Build history of the part. All positions in model axes, mm. A direction names the side the tool comes from. Give positions to 0.01 mm unless a question says otherwise; leave off trailing zeros. Write each loop counter-clockwise with the first axis right and the second up, starting at its lowest first coordinate (ties: lowest second). Pieces come first, ordered by that corner, then holes. Notation, with made-up numbers: (55.25, 47) -> (99.25, 47) arc R16 ccw to (99.25, 61) -> close; hole circle Ø11 at (-6, 75). An arc over 180 degrees is marked (long way). One line per question, with ' | ' between items. Start each with the question number.
(1) Tool access for faces 1 (the cylindrical face through (4.93, 9.352, -9.474)), 2 (the flat face through (0, 0.2, -3.3)): list every direction of +Z, -Z, +X, -X, +Y, -Y with a clear straight run to the whole face (end or side of a thin tool).
(2) Band-saw the part on C-C, the plane x = 86.5. Give the cut face in (y, z).
(3) Drill centre lines: probe 1 along Y at (x, z) = (6.25, -8); probe 2 along Y at (x, z) = (0.7, 0); probe 3 along X at (y, z) = (8.5, -14). Where is each one in solid material? Low to high. Write a range as from..to.
(4) Pin check, flat tips, straight feed: P1, Ø5, axis at x = 73.5, y = -7.5, coming from the -Z side; P2, Ø10, axis at x = 72, z = -0.5, coming from the -Y side; P3, Ø1.5, axis at x = 111.5, y = 2.5, coming from the +Z side; P4, Ø1.5, axis at y = -15, z = -14, coming from the -X side. Stop position of each tip, or through.
(5) Pull direction Z, two halves, no side cores. Call faces 3 (the flat face through (123.8, 0, 0)), 4 (the flat face through (10, -8, -8)), 5 (the cylindrical face through (87.16, 18.59, 2.44)): released by +Z, released by -Z, zero draft, split by the parting line, or undercut.
from build123d import *

# Parameters (mm, degrees)
SKETCH2_R           = 16
BOSS_EXTRUDE1_DEPTH = 48.8
SKETCH3_R           = 18.75
BOSS_EXTRUDE2_DEPTH = 75
FILLET1_R           = 2.74
SKETCH4_R           = 3
CUT_EXTRUDE1_DEPTH  = 2
SKETCH5_R           = 2
CUT_EXTRUDE2_DEPTH  = 10


with BuildPart() as part:
    # Sketch2 → Boss-Extrude1 (new body)
    with BuildSketch(Plane(origin=(0, 0, 0), x_dir=(0, 0, -1), z_dir=(1, 0, 0))):
        Circle(SKETCH2_R)
    extrude(amount=BOSS_EXTRUDE1_DEPTH)

    # Sketch3 → Boss-Extrude2 (add)
    with BuildSketch(Plane(origin=(48.8, 0, 0), x_dir=(0, 0, -1), z_dir=(1, 0, 0))):
        Circle(SKETCH3_R)
    extrude(amount=BOSS_EXTRUDE2_DEPTH)

    # Fillet1
    fillet1_edges = [part.edges().sort_by_distance(p)[0] for p in [
        (48.8, 0, 18.75),
    ]]
    fillet(fillet1_edges, radius=FILLET1_R)

    # Sketch4 → Cut-Extrude1 (cut)
    with BuildSketch(Plane.ZY):
        Circle(SKETCH4_R)
    extrude(amount=-CUT_EXTRUDE1_DEPTH, mode=Mode.SUBTRACT)

    # Sketch5 → Cut-Extrude2 (cut)
    with BuildSketch(Plane.ZY):
        with Locations((-8, 8)):
            Circle(SKETCH5_R)
        with Locations(Location((8, 8, 0), (0, 0, 180))):
            Circle(SKETCH5_R)
        with Locations((8, -8)):
            Circle(SKETCH5_R)
        with Locations(Location((-8, -8, 0), (0, 0, 180))):
            Circle(SKETCH5_R)
    extrude(amount=-CUT_EXTRUDE2_DEPTH, mode=Mode.SUBTRACT)


solid = part.part
Results:
1) face 1: -X | face 2: +Z, -Z, -X, +Y, -Y
2) outline: circle Ø37.5 at (0, 0)
3) probe 1: y = -13.86..-10, -6..6, 10..13.86 | probe 2: y = -16..-3, 3..16 | probe 3: x = 48.82..123.8
4) P1: stops at z = -18.07 | P2: stops at y = -18.75 | P3: stops at z = 18.67 | P4: passes through
5) face 3: zero draft | face 4: undercut | face 5: split by the parting line
